```python
from build123d import *

# Parameters (mm, degrees)
F2_R     = 7.5
F3_DEPTH = 44
F5_START = 11.37151
F4_R     = 3
F4_R_2   = 5
F5_DEPTH = 8.99461


with BuildPart() as f1:
    # F0 (on Front) → F1 (revolve)
    with BuildSketch(Plane.XZ):
        with BuildLine():
            Line((7, 44), (0, 44))
            Line((0, 44), (0, 0))
            Line((0, 0), (12, 0))
            Line((12, 0), (12, 3))
            Line((12, 3), (13, 3))
            ThreePointArc((13, 3), (16.5355339059, 4.4644660941), (18, 8))
            Line((18, 8), (18, 31))
            ThreePointArc((18, 31), (16.5355339059, 34.5355339059), (13, 36))
            Line((13, 36), (9, 36))
            Line((9, 36), (9, 42))
            ThreePointArc((9, 42), (8.4142135624, 43.4142135624), (7, 44))
        make_face()
    revolve(axis=Axis((0, 0, 22), (0, 0, 1)))

    # F2 (on face) → F3 (cut, through all)
    with BuildSketch(Plane(origin=(0, 0, 0), x_dir=(1, 0, 0), z_dir=(0, 0, -1))):
        Circle(F2_R)
    extrude(amount=-F3_DEPTH, mode=Mode.SUBTRACT)

    # F4 (on Front) → F5 (cut)
    with BuildSketch(Plane.XZ.offset(F5_START)):
        with Locations((7, 25)):
            Circle(F4_R)
        with Locations((-7, 25)):
            Circle(F4_R_2)
    extrude(amount=F5_DEPTH, mode=Mode.SUBTRACT)


solid = f1.part
```
For this review, take the finished solid that the model builds, in its own axes (mm). A direction names the side the tool comes from. Round coordinates to 2 decimals unless told otherwise and drop trailing zeros. Write each loop counter-clockwise with the first axis right and the second up, starting at its lowest first coordinate (ties: lowest second). Pieces come first, ordered by that corner, then holes. Notation, with made-up numbers: M 31,89.5 L 89,89.5 A19 cw 89,102.5 Z; hole C -38.5,29 d10. An arc over 180 degrees is marked long. One line per item, written item: value. Start each with the question number.
(1) We need section A-A (x = 0). Give the boundary of the cut face in (y, z), and give its area (3 significant figures).
(2) We need section C-C (z = 39.5). Give the boundary of the cut face in (x, y), and give its area (3 significant figures).
(3) Insertion check: pin 1 (10 mm diameter, centred on x = 7, z = 39, fed in from +Y); pin 2 (5 mm diameter, centred on x = 7, z = 25, fed in from -Y); pin 3 (6 mm diameter, centred on y = 4.5, z = 18, fed in from +X); pin 4 (13 mm diameter, centred on x = 5, y = -5, fed in from -Z). Each pin has a flat end and moves straight along its axis. Give the tip position at first contact, or say it passes through.
(4) The part is to be moulded in two halves that separate along X. For faces 4 (the cylindrical face through (-11.99, 0.53, 1.52)), 5 (the cylindrical face through (4, -14, 25)), 6 (the flat face through (3, 9, 36)), say which applies: released by +X, released by -X, zero draft, split by the parting line, or undercut.
(5) We need section B-B (z = 26). Give the boundary of the cut face in (x, y).
(6) Wall thickness on line 1 (Y direction, x = 0, z = 23); line 2 (X direction, y = -13, z = 26); line 3 (Z direction, x = -6, y = -12): over which ranges is each line inside the solid? List them lowest first.
(7) Machinability: for faces 1 (the flat face through (-7, -11.372, 25)), 2 (the cylindrical face through (-1.172, 8.923, 39.042)), 3 (the flat face through (-9, -9, 3)), which of the approach directions +Z, -Z, +X, -X, +Y, -Y give a long, thin tool a straight path to every point of the face, cutting with its end or side? Answer none if there is none.
(8) We need section D-D (z = 12). Give the boundary of the cut face in (x, y), and give its area (3 significant figures).
Result:
1. outline: M -18,8 A5 ccw -13,3 L -12,3 L -12,0 L -7.5,0 L -7.5,43.94 A2 ccw -9,42 L -9,36 L -13,36 A5 ccw -18,31 Z; M 7.5,0 L 12,0 L 12,3 L 13,3 A5 ccw 18,8 L 18,31 A5 ccw 13,36 L 9,36 L 9,42 A2 ccw 7.5,43.94 Z
1. area: 721 mm²
2. outline: C 0,0 d18; hole C 0,0 d15
2. area: 77.8 mm²
3. pin 1: y = 15.9
3. pin 2: y = -11.37
3. pin 3: x = 17.94
3. pin 4: z = 0
4. face 4: split by the parting line
4. face 5: undercut
4. face 6: zero draft
5. outline: M -11.9,-13.51 L -11.9,-11.37 L -2.1,-11.37 L -2.1,-17.88 A18 ccw 4.17,-17.51 L 4.17,-11.37 L 9.83,-11.37 L 9.83,-15.08 A18 ccw long Z; hole C 0,0 d15
6. line 1: -18 to -7.5, 7.5 to 18
6. line 2: -12.45 to -11.9, -2.1 to 4.17, 9.83 to 12.45
6. line 3: 3.02 to 20.1, 29.9 to 35.98
7. face 1: -Y
7. face 2: +Z
7. face 3: -Z
8. outline: C 0,0 d36; hole C 0,0 d15
8. area: 841 mm²
